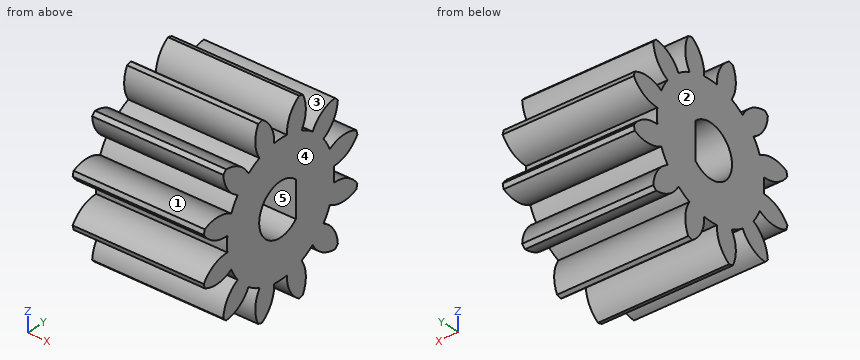
```python
from build123d import *

# Parameters (mm, degrees)
BASPROSKE_W        = 12
BASPROSKE_H        = 8.75
TOOTHCUT_DEPTH     = 18.237314176
TEETHCUTS_COUNT    = 12
TEETHCUTS_ANGLE    = 330
BORSKE_R           = 0.4
BORE_DEPTH         = 50.0000508
CUT_EXTRUDE1_DEPTH = 17.991923373


with BuildPart() as part:
    # BasProSke → Base-Revolve (revolve)
    with BuildSketch(Plane(origin=(0, 0, 0), x_dir=(1, 0, 0), z_dir=(0, 1, 0)), mode=Mode.PRIVATE) as base_revolve_sk:
        with Locations((6, 4.375)):
            Rectangle(BASPROSKE_W, BASPROSKE_H)
    revolve(base_revolve_sk.sketch.rotate(Axis((-10, 0, 0), (1, 0, 0)), 180), axis=Axis((-10, 0, 0), (1, 0, 0)))

    # TooCutSke → ToothCut (cut, through all)
    with BuildSketch(Plane(origin=(0, 0, 0), x_dir=(0, 0, -1), z_dir=(1, 0, 0))):
        with BuildLine():
            ThreePointArc((0.699286786, 5.895170077), (0, 5.9365), (-0.699286786, 5.895170077))
            ThreePointArc((-0.699286786, 5.895170077), (-1.040581249, 7.393099844), (-2.078649209, 8.525659073))
            ThreePointArc((-2.078649209, 8.525659073), (0, 8.7754), (2.078649209, 8.525659073))
            ThreePointArc((2.078649209, 8.525659073), (1.040581249, 7.393099844), (0.699286786, 5.895170077))
        make_face()
    toothcut = extrude(amount=TOOTHCUT_DEPTH, mode=Mode.SUBTRACT)

    # TeethCuts: ToothCut ×12 about axis
    teethcuts_axis = Axis((-10, 0, 0), (1, 0, 0))
    for i in range(1, TEETHCUTS_COUNT):
        add(toothcut.rotate(teethcuts_axis, i * TEETHCUTS_ANGLE / (TEETHCUTS_COUNT - 1)), mode=Mode.SUBTRACT)

    # BorSke → Bore (cut, symmetric)
    with BuildSketch(Plane(origin=(0, 0, 0), x_dir=(0, 0, -1), z_dir=(1, 0, 0))):
        with Locations(Location((0, 0, 0), (0, 0, 180))):
            Circle(BORSKE_R)
    extrude(amount=BORE_DEPTH, both=True, mode=Mode.SUBTRACT)

    # Sketch1 → Cut-Extrude1 (cut, through all)
    with BuildSketch(Plane(origin=(12, 0, 0), x_dir=(0, 0, -1), z_dir=(1, 0, 0))):
        with BuildLine():
            Line((-1.661565527, 1.69), (1.661565527, 1.69))
            ThreePointArc((1.661565527, 1.69), (0, -2.37), (-1.661565527, 1.69))
        make_face()
    extrude(amount=-CUT_EXTRUDE1_DEPTH, mode=Mode.SUBTRACT)


solid = part.part
```
Input: part model. Units: mm. Frame: model coordinates. Face numbers are marked on the shaded views. A direction names the side the tool comes from. Give positions to 0.01 mm unless a question says otherwise; leave off trailing zeros. Order: outer loops, then holes, each group sorted by start corner. A loop starts at its lowest first (then second) coordinate and runs counter-clockwise, first axis right, second up. Notation, with made-up numbers: (-35.5, 74) - (11.5, 74) arc R13 cw to (11.5, 86) - close; hole circle Ø9 at (-17, 68.5). An arc over 180 degrees is marked (long way). Use a Markdown table: item, result.
(1) Line query: line 1 (Y direction, x = 3, z = 0); line 2 (Z direction, x = 7, y = -6); line 3 (Z direction, x = 4.5, y = 0). Output: solid intervals per line, ascending. Write a range as from..to.
Computed values:
| item | result |
|---|---|
| line 1 | y = -5.94..-2.37, 1.69..5.94 |
| line 2 | z = -6.34..-4.8, -2.61..-0.7, 0.7..2.61, 4.8..6.34 |
| line 3 | z = -5.94..-2.37, 2.37..5.94 |
(2) Section query A-A (z = 0). Output: boundary loops of the cut face in (x, y), then the cut area to 3 significant figures.
Computed values:
| item | result |
|---|---|
| outline | (0, -5.94) - (12, -5.94) - (12, -2.37) - (0, -2.37) - close; (0, 1.69) - (12, 1.69) - (12, 5.94) - (0, 5.94) - close |
| area | 93.8 mm2 |
(3) Draft query along Y for the marked faces 1 and 2. Return one class per face: released by +Y, released by -Y, zero draft, split by the parting line, or undercut.
Computed values:
| item | result |
|---|---|
| face 1 | undercut |
| face 2 | zero draft |
(4) Section query B-B (y = 0). Output: boundary loops of the cut face in (x, z).
Computed values:
| item | result |
|---|---|
| outline | (0, -5.94) - (12, -5.94) - (12, -2.37) - (0, -2.37) - close; (0, 2.37) - (12, 2.37) - (12, 5.94) - (0, 5.94) - close |
(5) Access query for the marked faces 3, 4 and 5. Directions: +Z, -Z, +X, -X, +Y, -Y. A direction counts if a zero-diameter tool reaches every point of the face in a straight line with its end or side. Return the directions, or none.
Computed values:
| item | result |
|---|---|
| face 3 | +Z, +X, -X |
| face 4 | +Z, -Z, +X, +Y, -Y |
| face 5 | +X, -X |
(6) Pin query (flat end, axial travel): pin 1 (1 mm diameter, centred on x = 5.5, z = -6.5, fed in from -Y); pin 2 (1.5 mm diameter, centred on x = 5.5, z = -5, fed in from +Y); pin 3 (2 mm diameter, centred on x = 8, y = -1, fed in from -Z). Return the tip coordinate at first contact, or that it passes through.
Computed values:
| item | result |
|---|---|
| pin 1 | stops at y = -6.34 |
| pin 2 | stops at y = 6.31 |
| pin 3 | stops at z = -8.47 |
(7) Section query C-C (y = -3.25). Output: boundary loops of the cut face in (x, z).
Computed values:
| item | result |
|---|---|
| outline | (0, -4.97) - (12, -4.97) - (12, 4.97) - (0, 4.97) - close |
